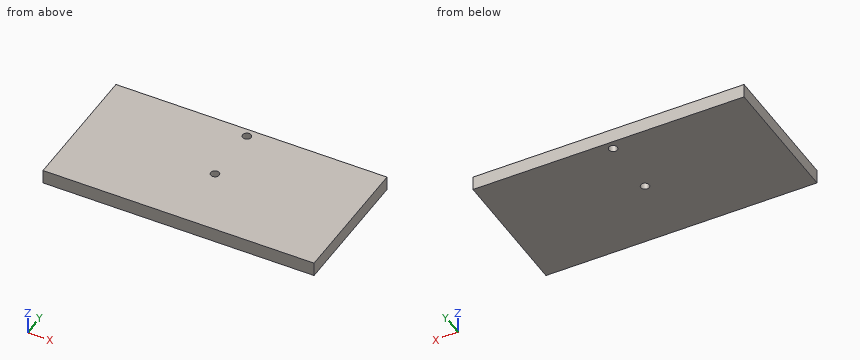
from build123d import *

# Parameters (mm, degrees)
F0_W     = 1219.2
F0_H     = 63.5
F1_DEPTH = 304.8
F2_R     = 19.05
F3_DEPTH = 63.501
F4_R     = 19.05
F5_DEPTH = 63.501


with BuildPart() as f1:
    # F0 (on Front) → F1 (new body, symmetric)
    with BuildSketch(Plane.XZ):
        Rectangle(F0_W, F0_H)
    extrude(amount=F1_DEPTH, both=True)

    # F2 (on face) → F3 (cut, through all)
    with BuildSketch(Plane.XY.offset(31.75)):
        Circle(F2_R)
    extrude(amount=-F3_DEPTH, mode=Mode.SUBTRACT)

    # F4 (on face) → F5 (cut, through all)
    with BuildSketch(Plane.XY.offset(31.75)):
        with Locations((0, 266.7)):
            Circle(F4_R)
    extrude(amount=-F5_DEPTH, mode=Mode.SUBTRACT)


solid = f1.part
The model under review builds one solid part; all positions refer to its coordinate system, in mm. Round coordinates to 2 decimals unless told otherwise and drop trailing zeros. Loops run counter-clockwise (first coordinate to the right, second up) from the corner with the lowest first, then second, coordinate; pieces in that order, holes last. Notation, with made-up numbers: M 32,4 L 77,4 A19 cw 77,24 Z; hole C 78,83 d10. An arc over 180 degrees is marked long. Answer as CSV lines item,"result".
1. We need section A-A (y = 266.7). Give the boundary of the cut face in (x, z).
Outcome:
outline,"M -609.6,-31.75 L -19.05,-31.75 L -19.05,31.75 L -609.6,31.75 Z; M 19.05,-31.75 L 609.6,-31.75 L 609.6,31.75 L 19.05,31.75 Z"
2. To check wall thickness, follow L1, parallel to Y at x = 0, z = -7; L2, parallel to X at y = 266, z = -10; L3, parallel to Y at x = -11, z = -6. State the ranges of each line that lie inside material, in increasing order. Write a range as [from, to].
Outcome:
L1,"y = [-304.8, -19.05], [19.05, 247.65], [285.75, 304.8]"
L2,"x = [-609.6, -19.04], [19.04, 609.6]"
L3,"y = [-304.8, -15.55], [15.55, 251.15], [282.25, 304.8]"
3. We need section B-B (x = 0). Give the boundary of the cut face in (y, z).
Outcome:
outline,"M -304.8,-31.75 L -19.05,-31.75 L -19.05,31.75 L -304.8,31.75 Z; M 19.05,-31.75 L 247.65,-31.75 L 247.65,31.75 L 19.05,31.75 Z; M 285.75,-31.75 L 304.8,-31.75 L 304.8,31.75 L 285.75,31.75 Z"
